Can you work these out from the drawing? Everything is in mm from the part's minimum corner. Round coordinates to 2 decimals unless told otherwise and drop trailing zeros. Write each loop counter-clockwise with the first axis right and the second up, starting at its lowest first coordinate (ties: lowest second). Pieces come first, ordered by that corner, then holes. Notation, with made-up numbers: (-26.5, -36.5) -> (-0.5, -36.5) arc R27 cw to (-0.5, -8.5) -> close; hole circle Ø2 at (-29, 67). An arc over 180 degrees is marked (long way). Answer as CSV lines item,"result". Start each with the question number.
Q1. If I drill on line 1 (Z direction, x = 10, y = 29); line 2 (X direction, y = 29.35, z = 10); line 3 (Y direction, x = 10, z = 18), over which ranges is the centre line in solid material (lowest first)? Write a range as [from, to].
Q2. Imagine slicing it at D-D on z = 10. Please give me the cut outline in (x, y).
Q3. Imagine slicing it at A-A on x = 70. Please give me the cut outline in (y, z).
Q4. If we mould it in two halves opening along X, with no side actions, what happens to the marked faces 1, 2 and 3? For each: pulls with the +X half, pulls with the -X half, needs draft (parallel to the pull), parting line crosses it, or undercut.
Q5. Imagine slicing it at B-B on y = 16. Please give me the cut outline in (x, z), and give its area (3 significant figures).
Q6. Imagine slicing it at C-C on z = 21.5. Please give me the cut outline in (x, y), and give its area (3 significant figures).
Q7. Will this pin go through, and if not, where does the flat tip stop? pin 1 Ø1.6 at (x, z) = (11, 10.5) entering from +Y.
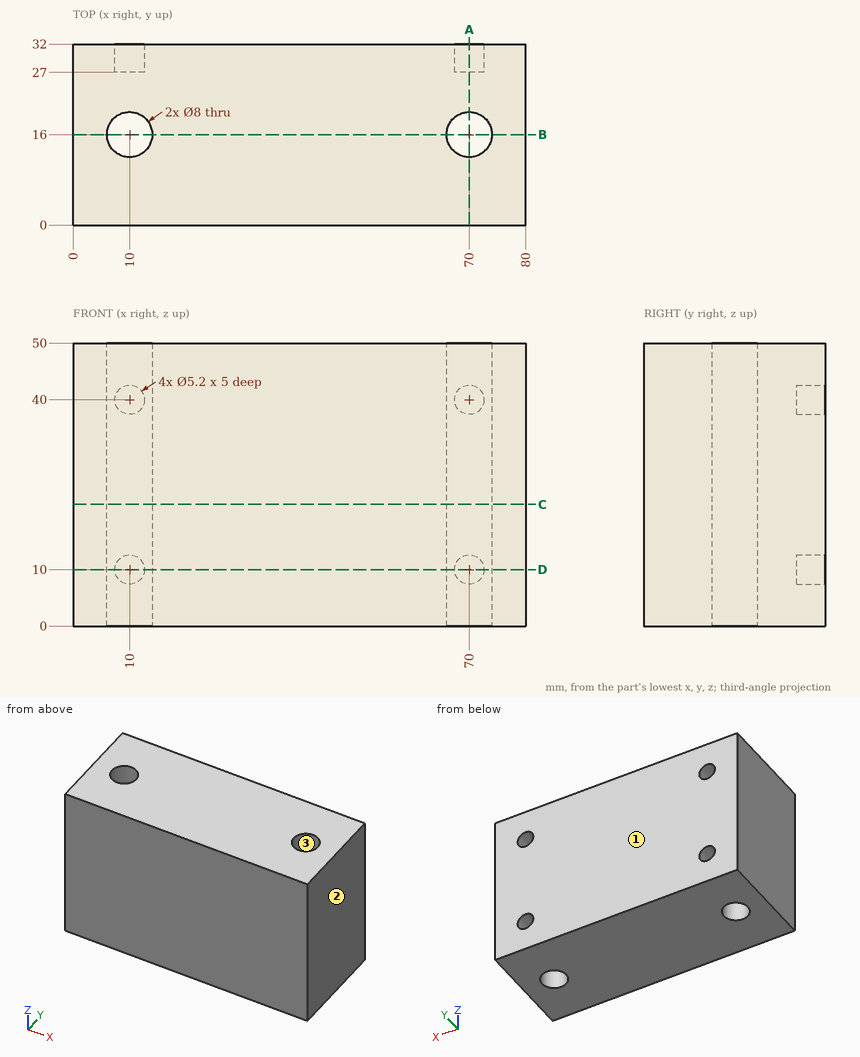
Checks:
1,line 1,"[0, 7.4], [12.6, 37.4], [42.6, 50]"
1,line 2,"[0, 7.4], [12.6, 67.4], [72.6, 80]"
1,line 3,"[0, 12], [20, 32]"
2,outline,"(0, 0) -> (80, 0) -> (80, 32) -> (72.6, 32) -> (72.6, 27) -> (67.4, 27) -> (67.4, 32) -> (12.6, 32) -> (12.6, 27) -> (7.4, 27) -> (7.4, 32) -> (0, 32) -> close; hole circle Ø8 at (10, 16); hole circle Ø8 at (70, 16)"
3,outline,"(0, 0) -> (12, 0) -> (12, 50) -> (0, 50) -> close; (20, 0) -> (32, 0) -> (32, 7.4) -> (27, 7.4) -> (27, 12.6) -> (32, 12.6) -> (32, 37.4) -> (27, 37.4) -> (27, 42.6) -> (32, 42.6) -> (32, 50) -> (20, 50) -> close"
4,face 1,"needs draft"
4,face 2,"pulls with the +X half"
4,face 3,"undercut"
5,outline,"(0, 0) -> (6, 0) -> (6, 50) -> (0, 50) -> close; (14, 0) -> (66, 0) -> (66, 50) -> (14, 50) -> close; (74, 0) -> (80, 0) -> (80, 50) -> (74, 50) -> close"
5,area,"3,200 mm^2"
6,outline,"(0, 0) -> (80, 0) -> (80, 32) -> (0, 32) -> close; hole circle Ø8 at (10, 16); hole circle Ø8 at (70, 16)"
6,area,"2,460 mm^2"
7,pin 1,"y = 27"
